Geometry: final body of the model. Coordinates: model frame, mm. A direction names the side the tool comes from. Give positions to 0.01 mm unless a question says otherwise; leave off trailing zeros. Loops run counter-clockwise (first coordinate to the right, second up) from the corner with the lowest first, then second, coordinate; pieces in that order, holes last. Notation, with made-up numbers: M 61,53 L 115,53 A8 cw 115,57 Z; hole C -29.5,-16 d2. An arc over 180 degrees is marked long. Put each result on its own line as item: value.
```python
from build123d import *

# Parameters (mm, degrees)
SKETCH1_W           = 98
SKETCH1_H           = 98
BOSS_EXTRUDE1_DEPTH = 18
SKETCH2_W           = 24
SKETCH2_H           = 13.1
CUT_EXTRUDE1_DEPTH  = 18
SKETCH2_4_W         = 5.2
SKETCH2_4_H         = 12.7
SKETCH2_4_H_2       = 0.2
CUT_EXTRUDE2_DEPTH  = 10
CUT_EXTRUDE3_DEPTH  = 8
SKETCH5_W           = 10
SKETCH5_H           = 5
CUT_EXTRUDE4_DEPTH  = 18
SKETCH6_W           = 5
SKETCH6_H           = 20
BOSS_EXTRUDE2_DEPTH = 16
FILLET1_R           = 1
FILLET2_R           = 1
CUT_EXTRUDE5_DEPTH  = 18


with BuildPart() as part:
    # Sketch1 → Boss-Extrude1 (new body)
    with BuildSketch(Plane.XY):
        Rectangle(SKETCH1_W, SKETCH1_H)
    extrude(amount=BOSS_EXTRUDE1_DEPTH)

    # Sketch2 → Cut-Extrude1 (cut)
    with BuildSketch(Plane(origin=(0, 0, 0), x_dir=(-1, 0, 0), z_dir=(0, 0, -1))):
        with Locations((-5.65, 0)):
            Rectangle(SKETCH2_W, SKETCH2_H)
    extrude(amount=-CUT_EXTRUDE1_DEPTH, mode=Mode.SUBTRACT)

    # Sketch2<4> → Cut-Extrude2 (cut)
    with BuildSketch(Plane(origin=(0, 0, 0), x_dir=(-1, 0, 0), z_dir=(0, 0, -1))):
        with Locations((-20.25, 0)):
            Rectangle(SKETCH2_4_W, SKETCH2_4_H)
        Polygon((-22.85, 6.35), (-17.65, 6.35), (-17.65, 6.55), (-22.85, 6.55), (-23.05, 6.55), (-23.05, 6.35), (-23.05, -6.55), (-17.65, -6.55), (-17.65, -6.35), (-22.85, -6.35), align=None)
        Polygon((11.55, 6.35), (6.35, 6.35), (6.35, 0), (6.35, -6.15), (11.55, -6.15), align=None)
        Polygon((6.35, 6.55), (6.35, 6.35), (11.55, 6.35), (11.55, -6.15), (11.55, -6.35), (6.35, -6.35), (6.35, -6.55), (11.55, -6.55), (11.75, -6.55), (11.75, -6.35), (11.75, 6.55), align=None)
        with Locations((8.95, -6.25)):
            Rectangle(SKETCH2_4_W, SKETCH2_4_H_2)
    extrude(amount=-CUT_EXTRUDE2_DEPTH, mode=Mode.SUBTRACT)

    # Sketch4 → Cut-Extrude3 (cut)
    with BuildSketch(Plane(origin=(0, 0, 10), x_dir=(-1, 0, 0), z_dir=(0, 0, -1))):
        Polygon((6.35, 0), (6.35, 2.5), (9.35, 2.5), (9.35, -2.5), (6.35, -2.5), align=None)
    extrude(amount=-CUT_EXTRUDE3_DEPTH, mode=Mode.SUBTRACT)

    # Sketch5 → Cut-Extrude4 (cut)
    with BuildSketch(Plane.XY.offset(18)):
        with Locations((-14.35, 0)):
            Rectangle(SKETCH5_W, SKETCH5_H)
        Polygon((-19.35, 2.5), (-9.35, 2.5), (-9.35, 19), (8, 19), (8, 29), (8, 49), (0, 49), (-8, 49), (-8, 29), (-19.35, 29), align=None)
        Polygon((-9.35, -19), (-9.35, -2.5), (-19.35, -2.5), (-19.35, -29), (-8, -29), (-8, -49), (0, -49), (8, -49), (8, -29), (8, -19), align=None)
    extrude(amount=-CUT_EXTRUDE4_DEPTH, mode=Mode.SUBTRACT)


with BuildPart() as cut_extrude4_piece_1:
    # of the separate pieces the step leaves, piece 1, a body of its own (cut_extrude4_pieces)
    add(part.part.solids().sort_by_distance((8, 49, 0))[0])



with BuildPart() as cut_extrude4_piece_2:
    # of the separate pieces the step leaves, piece 2, a body of its own (cut_extrude4_pieces)
    add(part.part.solids().sort_by_distance((-49, 49, 0))[0])


with BuildPart() as cut_extrude4_piece_1_1:
    add(cut_extrude4_piece_1.part)

    add(cut_extrude4_piece_2.part)  # Boss-Extrude2 merges Cut-Extrude4 piece 2
    # Sketch6 → Boss-Extrude2 (add)
    with BuildSketch(Plane(origin=(-8, 0, 0), x_dir=(0, 0, -1), z_dir=(1, 0, 0))):
        with Locations((-15.5, 39)):
            Rectangle(SKETCH6_W, SKETCH6_H)
        with Locations((-2.5, 39)):
            Rectangle(SKETCH6_W, SKETCH6_H)
        with Locations((-15.5, -39)):
            Rectangle(SKETCH6_W, SKETCH6_H)
        with Locations((-2.5, -39)):
            Rectangle(SKETCH6_W, SKETCH6_H)
    extrude(amount=BOSS_EXTRUDE2_DEPTH)

    # Fillet1
    fillet1_edges = [cut_extrude4_piece_1_1.edges().sort_by_distance(p)[0] for p in [
        (-19.35, 0, 0),
        (-5.675, 29, 0),
        (-5.675, -29, 0),
        (-0.675, -19, 0),
        (-9.35, -12.775, 0),
        (6.85, -6.55, 0),
        (6.85, 6.55, 0),
        (-9.35, 12.775, 0),
        (49, 0, 0),
        (23.05, 0, 0),
        (-0.675, 19, 0),
        (8, 24, 0),
        (8, -24, 0),
        (0, -49, 0),
        (-49, 0, 0),
        (0, 49, 0),
    ]]
    fillet(fillet1_edges, radius=FILLET1_R)

    # Fillet2
    # the kernel refuses this fillet: 1 mm, written as the material it takes off along each edge
    with BuildSketch(Plane(origin=(48, -48, 1), x_dir=(0, -1, 0), z_dir=(1, 0, 0))) as fillet2_piece_1_section:
        Polygon((0, 0), (FILLET2_R, 0), (FILLET2_R, FILLET2_R), (0, FILLET2_R), align=None)
    fillet2_piece_1 = extrude(amount=FILLET2_R, mode=Mode.PRIVATE)
    fillet2_piece_1 = fillet2_piece_1 - Plane(origin=(48, -48, 1), x_dir=(0, 0.7071067811865475, 0.7071067811865475), z_dir=(1, 0, 0)) * Sphere(FILLET2_R, mode=Mode.PRIVATE)
    add(fillet2_piece_1, mode=Mode.SUBTRACT)
    with BuildSketch(Plane(origin=(-48, -48, 1), x_dir=(0, -1, 0), z_dir=(-1, 0, 0))) as fillet2_piece_2_section:
        Polygon((0, 0), (FILLET2_R, 0), (FILLET2_R, -FILLET2_R), (0, -FILLET2_R), align=None)
    fillet2_piece_2 = extrude(amount=FILLET2_R, mode=Mode.PRIVATE)
    fillet2_piece_2 = fillet2_piece_2 - Plane(origin=(-48, -48, 1), x_dir=(0, 0.7071067811865475, 0.7071067811865475), z_dir=(-1, 0, 0)) * Sphere(FILLET2_R, mode=Mode.PRIVATE)
    add(fillet2_piece_2, mode=Mode.SUBTRACT)
    with BuildSketch(Plane(origin=(48, 48, 1), x_dir=(1, 0, 0), z_dir=(0, 1, 0))) as fillet2_piece_3_section:
        Polygon((0, 0), (FILLET2_R, 0), (FILLET2_R, FILLET2_R), (0, FILLET2_R), align=None)
    fillet2_piece_3 = extrude(amount=FILLET2_R, mode=Mode.PRIVATE)
    fillet2_piece_3 = fillet2_piece_3 - Plane(origin=(48, 48, 1), x_dir=(-0.7071067811865475, 0, 0.7071067811865475), z_dir=(0, 1, 0)) * Sphere(FILLET2_R, mode=Mode.PRIVATE)
    add(fillet2_piece_3, mode=Mode.SUBTRACT)
    with BuildSketch(Plane(origin=(-48, 48, 1), x_dir=(-1, 0, 0), z_dir=(0, 1, 0))) as fillet2_piece_4_section:
        Polygon((0, 0), (FILLET2_R, 0), (FILLET2_R, -FILLET2_R), (0, -FILLET2_R), align=None)
    fillet2_piece_4 = extrude(amount=FILLET2_R, mode=Mode.PRIVATE)
    fillet2_piece_4 = fillet2_piece_4 - Plane(origin=(-48, 48, 1), x_dir=(0.7071067811865475, 0, 0.7071067811865475), z_dir=(0, 1, 0)) * Sphere(FILLET2_R, mode=Mode.PRIVATE)
    add(fillet2_piece_4, mode=Mode.SUBTRACT)
    with BuildSketch(Plane(origin=(49, 49, 1), x_dir=(-1, 0, 0), z_dir=(0, 0, 1)), Plane(origin=(49, -49, 1), x_dir=(0, 1, 0), z_dir=(0, 0, 1))) as fillet2_piece_5:
        with BuildLine():
            CenterArc((FILLET2_R, FILLET2_R), FILLET2_R, 180, 90)
            Line((0, FILLET2_R), (0, 0))
            Line((0, 0), (FILLET2_R, 0))
        make_face()
    extrude(amount=19.5, mode=Mode.SUBTRACT)
    with BuildSketch(Plane(origin=(-49, -49, 1), x_dir=(0, 1, 0), z_dir=(0, 0, 1)), Plane(origin=(-49, 49, 1), x_dir=(1, 0, 0), z_dir=(0, 0, 1))) as fillet2_piece_6:
        with BuildLine():
            CenterArc((FILLET2_R, -FILLET2_R), FILLET2_R, 90, 90)
            Line((0, -FILLET2_R), (0, 0))
            Line((0, 0), (FILLET2_R, 0))
        make_face()
    extrude(amount=19.5, mode=Mode.SUBTRACT)

    # Sketch8 → Cut-Extrude5 (cut)
    with BuildSketch(Plane.XY.offset(18)):
        Polygon((-15, -34), (-34, -34), (-34, 34), (-15, 34), (-15, 44), (-44, 44), (-44, -44), (-15, -44), align=None)
        Polygon((34, -34), (15, -34), (15, -44), (44, -44), (44, 44), (15, 44), (15, 34), (34, 34), align=None)
    extrude(amount=-CUT_EXTRUDE5_DEPTH, mode=Mode.SUBTRACT)


solid = cut_extrude4_piece_1_1.part
```
Item 1: Pin query (flat end, axial travel): pin 1 Ø3.5 at (x, y) = (-8, -4.5) entering from -Z; pin 2 Ø1 at (x, y) = (17, -1.5) entering from +Z. Return the tip coordinate at first contact, or that it passes through.
Output values:
pin 1: z = 10
pin 2: through
Item 2: Line query: probe 1 along Y at (x, z) = (19, 4.5); probe 2 along X at (y, z) = (21, 13.25); probe 3 along X at (y, z) = (-6.5, 10.25). Output: solid intervals per line, ascending. Write a range as [from, to].
Output values:
probe 1: [-49, -44], [-34, -6.55], [6.55, 34], [44, 49]
probe 2: [-49, -44], [-34, -19.35], [8, 34], [44, 49]
probe 3: [-49, -44], [-34, -19.35], [-9.35, -6.35], [17.65, 34], [44, 49]
Item 3: Section A-A on y = -41.5. Output: boundary loops of the cut face in (x, z), then the cut area to 3 significant figures.
Output values:
outline: M -49,1 A1 ccw -48,0 L -44,0 L -44,18 L -49,18 Z; M -15,0 L 15,0 L 15,18 L -15,18 Z; M 44,0 L 48,0 A1 ccw 49,1 L 49,18 L 44,18 Z; hole M -8,5 L 8,5 L 8,13 L -8,13 Z
area: 592 mm²
Item 4: Set-up query: faces 3 (the flat face through (-49, -1, 9)), 4 (the flat face through (-8, 39, 9)), 5 (the flat face through (24, 34, 9)), 6 (the flat face through (0, -39, 5)), 7 (the flat face through (7, 6.55, 9)). Return all of +Z, -Z, +X, -X, +Y, -Y with unobstructed straight access to the full face (end or side cutting, diameter ignored); none if empty.
Output values:
face 3: +Z, -Z, -X, +Y, -Y
face 4: +Y
face 5: +Z, -Z
face 6: -Y
face 7: -Z
Item 5: Section C-C on y = -4. Output: boundary loops of the cut face in (x, z), then the cut area to 3 significant figures.
Output values:
outline: M -49,1 A1 ccw -48,0 L -44,0 L -44,18 L -49,18 Z; M -34,0 L -20.35,0 A1 ccw -19.35,1 L -19.35,18 L -34,18 Z; M -9.35,10 L -6.35,10 L -6.35,18 L -9.35,18 Z; M 17.65,10 L 23.05,10 L 23.05,1 A1 ccw 24.05,0 L 34,0 L 34,18 L 17.65,18 Z; M 44,0 L 48,0 A1 ccw 49,1 L 49,18 L 44,18 Z
area: 707 mm²
Item 6: Mould query, pull axis Z, two halves, no side actions, for faces 1 (the flat face through (8, 30, 10)), 2 (the flat face through (-8, -2.5, 14)). Classes: pulls with the +Z half, pulls with the -Z half, needs draft (parallel to the pull), parting line crosses it, or undercut.
Output values:
face 1: undercut
face 2: needs draft
Item 7: Section D-D on x = 0. Count the separate pieces of the cut face and the enclosed holes in it, then the cut area to 3 significant figures.
Output values:
separate pieces: 6
enclosed holes: 0
area: 846 mm²
Item 8: Section B-B on x = 36. Output: boundary loops of the cut face in (y, z), then the cut area to 3 significant figures.
Output values:
outline: M -49,1 A1 ccw -48,0 L -44,0 L -44,18 L -49,18 Z; M 44,0 L 48,0 A1 ccw 49,1 L 49,18 L 44,18 Z
area: 180 mm²
